from build123d import *

# Parameters (mm, degrees)
BOSS_EXTRUDE1_DEPTH                              = 5
BOSS_EXTRUDE1_START                              = 0.002576877
BOSS_EXTRUDE1_3_OUTLINE_W                        = 16
BOSS_EXTRUDE1_3_OUTLINE_H                        = 16
BOSS_EXTRUDE1_3_DEPTH                            = 0.997423124
SKETCH2_W                                        = 5.5
SKETCH2_H                                        = 12
CBORE_FOR_M3_HEX_HEAD_MACHINE_SCREW1_D           = 3.3
CBORE_FOR_M3_HEX_HEAD_MACHINE_SCREW1_DEPTH       = 18.260356386
CBORE_FOR_M3_HEX_HEAD_MACHINE_SCREW1_CBORE_D     = 5
CBORE_FOR_M3_HEX_HEAD_MACHINE_SCREW1_CBORE_DEPTH = 13.5
F_2_5_2_5_DIAMETER_HOLE1_D                       = 2.5
F_2_5_2_5_DIAMETER_HOLE1_DEPTH                   = 14.334936491
CHAMFER1_SIZE                                    = 0.2
CHAMFER2_SIZE                                    = 0.35


with BuildPart() as part:
    # Boss-Extrude1: read off the stored shape, not the designer's step
    # Boss-Extrude1 outline → Boss-Extrude1 (new body)
    with BuildSketch(Plane(origin=(0, 1, 0), x_dir=(-1, 0, 0), z_dir=(0, 1, 0))):
        Polygon((3.464101615, 6), (-3.464101615, 6), (-6.92820323, 0), (-3.464101615, -6), (3.464101615, -6), (6.92820323, 0), align=None)
    extrude(amount=BOSS_EXTRUDE1_DEPTH)

    # Boss-Extrude1 2 outline → Boss-Extrude1 2 (revolve)
    with BuildSketch(Plane.XY):
        with BuildLine():
            Line((0, 1.000000001), (0, 0))
            Line((0, 0), (5.92820323, 0))
            ThreePointArc((5.92820323, 0), (6.635310012, 0.292893219), (6.92820323, 1.000000001))
            Line((6.92820323, 1.000000001), (0, 1.000000001))
        make_face()
    revolve(axis=Axis((0, 0, 0), (0, 1, 0)))

    # Boss-Extrude1 3 outline → Boss-Extrude1 3 (cut)
    with BuildSketch(Plane(origin=(0, 0, 0), x_dir=(1, 0, 0), z_dir=(0, 1, 0)).offset(BOSS_EXTRUDE1_START)):
        Rectangle(BOSS_EXTRUDE1_3_OUTLINE_W, BOSS_EXTRUDE1_3_OUTLINE_H)
        Polygon((6.92820323, 0), (3.464101615, -6), (-3.464101615, -6), (-6.92820323, 0), (-3.464101615, 6), (3.464101615, 6), align=None, mode=Mode.SUBTRACT)
    extrude(amount=BOSS_EXTRUDE1_3_DEPTH, mode=Mode.SUBTRACT)

    # Sketch2 → Revolve1 (revolve)
    with BuildSketch(Plane.XY, mode=Mode.PRIVATE) as revolve1_sk:
        with Locations((2.75, 12)):
            Rectangle(SKETCH2_W, SKETCH2_H)
    revolve(revolve1_sk.sketch.rotate(Axis((0, 18, 0), (0, -1, 0)), 270), axis=Axis((0, 18, 0), (0, -1, 0)))

    # CBORE for M3 Hex Head Machine Screw1
    with Locations(Plane(origin=(0, 18, 0), x_dir=(1, 0, 0), z_dir=(0, 1, 0))):
        with Locations((0, 0)):
            CounterBoreHole(CBORE_FOR_M3_HEX_HEAD_MACHINE_SCREW1_D / 2, CBORE_FOR_M3_HEX_HEAD_MACHINE_SCREW1_CBORE_D / 2, CBORE_FOR_M3_HEX_HEAD_MACHINE_SCREW1_CBORE_DEPTH, depth=CBORE_FOR_M3_HEX_HEAD_MACHINE_SCREW1_DEPTH)

    # Ø2.5 (2.5) Diameter Hole1
    with Locations(Plane(origin=(2.75, 15, 4.763139721), x_dir=(0.866025403784, 0, -0.5), z_dir=(0.5, 0, 0.866025403784))):
        with Locations((0, 0)):
            Hole(F_2_5_2_5_DIAMETER_HOLE1_D / 2, depth=F_2_5_2_5_DIAMETER_HOLE1_DEPTH)

    # Chamfer1
    chamfer1_edges = [part.edges().sort_by_distance(p)[0] for p in [
        (-2.5, 18, 0),
    ]]
    chamfer(chamfer1_edges, length=CHAMFER1_SIZE)

    # Chamfer2
    chamfer2_edges = [part.edges().sort_by_distance(p)[0] for p in [
        (1.65, 0, 0),
    ]]
    chamfer(chamfer2_edges, length=CHAMFER2_SIZE)


solid = part.part
Work out the finished part from the listing and answer in its coordinate system (mm). A direction names the side the tool comes from. Give positions to 0.01 mm unless a question says otherwise; leave off trailing zeros. Loops run counter-clockwise (first coordinate to the right, second up) from the corner with the lowest first, then second, coordinate; pieces in that order, holes last. Notation, with made-up numbers: (12.5, 2.25) - (41.5, 2.25) arc R24 cw to (41.5, 28.25) - close; hole circle Ø8 at (16, 87). An arc over 180 degrees is marked (long way). Answer in a Markdown table with one row per item. Add a question column.
Q1. A tool of negligible diameter and unlimited length cuts with its end or side. For faces 4 (the cylindrical face through (-5.37, 12.08, 1.19)), 5 (the flat face through (3, 18, 1)), from which of +Z, -Z, +X, -X, +Y, -Y can it reach the whole face along a straight path? Write none if from no direction.
Q2. Determine the mould class of faces 1 (the flat face through (5.172, 2.959, -3.042)), 2 (the flat face through (-5.172, 2.959, 3.042)), 3 (the cylindrical face through (-0.85, 15.05, -3.97)) for opening direction X: released by +X, released by -X, zero draft, split by the parting line, or undercut.
Q3. The part is cut by section B-B (y = 15.75). Determine the outline of the cut face in (x, z), and give its area (3 significant figures).
Q4. The part is cut by section C-C (y = 8). Determine the outline of the cut face in (x, z), and give its area (3 significant figures).
Q5. The part is cut by section A-A (y = 4). Determine the outline of the cut face in (x, z).
Q6. Consider line 1 along Z through (x, y) = (0, 3.2); line 2 along X through (y, z) = (14.5, 0); line 3 along Y through (x, z) = (3, -5). Determine where each line is inside the solid, lowest interval first.
Q7. Each of these flat-tipped pins is pushed along its axis until it touches: P1, Ø1, axis at x = -2, y = 13, coming from the +Z side; P2, Ø4, axis at x = 0.5, y = 15, coming from the -Z side; P3, Ø1.5, axis at x = -1, z = 0, coming from the -Y side; P4, Ø2, axis at x = 0, z = 0, coming from the +Y side. Where does it stop, or does it pass through?
Solution:
| question | item | result |
|---|---|---|
| 1 | face 4 | +Y |
| 1 | face 5 | +Z, -Z, +X, -X, +Y |
| 2 | face 1 | released by +X |
| 2 | face 2 | released by -X |
| 2 | face 3 | undercut |
| 3 | outline | (-3.57, -4.18) - (-2.01, -1.48) arc R2.5 cw to (0.28, 2.48) - (1.84, 5.18) arc R5.5 ccw to start; (-1.84, -5.18) arc R5.5 ccw to (3.57, 4.18) - (2.01, 1.48) arc R2.5 cw to (-0.28, -2.48) - close |
| 3 | area | 63.2 mm² |
| 4 | outline | circle Ø11 at (0, 0); hole circle Ø5 at (0, 0) |
| 4 | area | 75.4 mm² |
| 5 | outline | (-6.93, 0) - (-3.46, -6) - (3.46, -6) - (6.93, 0) - (3.46, 6) - (-3.46, 6) - close; hole circle Ø3.3 at (0, 0) |
| 6 | line 1 | z = -6 to -1.65, 1.65 to 6 |
| 6 | line 2 | x = -5.5 to -2.5, 2.5 to 5.5 |
| 6 | line 3 | y = 0 to 6 |
| 7 | P1 | stops at z = 5.29 |
| 7 | P2 | stops at z = -5.5 |
| 7 | P3 | stops at y = 0.25 |
| 7 | P4 | passes through |
